The model under review builds one solid part; all positions refer to its coordinate system, in mm. Face numbers are marked on the shaded views. A direction names the side the tool comes from. Give positions to 0.01 mm unless a question says otherwise; leave off trailing zeros. Order: outer loops, then holes, each group sorted by start corner. A loop starts at its lowest first (then second) coordinate and runs counter-clockwise, first axis right, second up.
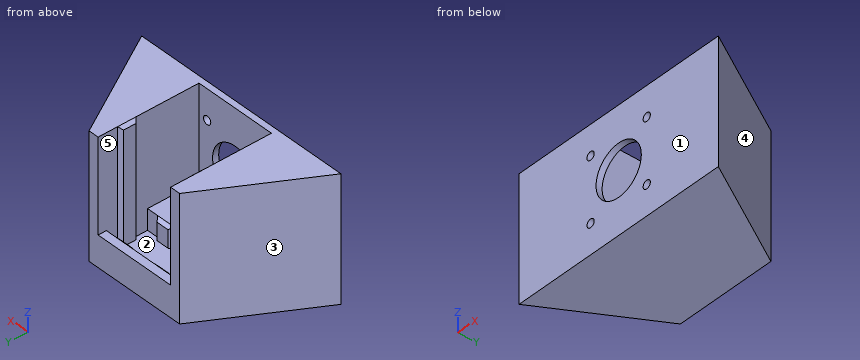
```python
from build123d import *

# Parameters (mm, degrees)
F1_DEPTH  = 60
F2_W      = 40
F2_H      = 20
F3_DEPTH  = 55
F4_W      = 40
F4_H      = 45
F5_DEPTH  = 4
F6_W      = 40
F6_H      = 45
F7_DEPTH  = 25
F8_R      = 12.5
F8_R_2    = 2
F9_DEPTH  = 2.9615242271
F10_W     = 9
F10_H     = 1.5
F10_W_2   = 1.5
F10_H_2   = 9
F11_DEPTH = 10
F12_DEPTH = 45
F13_SIZE  = 1.49999


# Not quite as in the source:
# - a fillet or chamfer is up to 0.001 mm smaller than in the source, because OpenCascade refuses the exact size


with BuildPart() as f1:
    # F0 (on Top) → F1 (new body)
    with BuildSketch(Plane.XY):
        Polygon((30, 51.9615242271), (0, 0), (110, 0), (80, 51.9615242271), align=None)
    extrude(amount=F1_DEPTH)

    # F2 (on face) → F3 (cut)
    with BuildSketch(Plane.XY.offset(60)):
        with Locations((55, 37.9615242271)):
            Rectangle(F2_W, F2_H)
    extrude(amount=-F3_DEPTH, mode=Mode.SUBTRACT)

    # F4 (on face) → F5 (cut, through all)
    with BuildSketch(Plane(origin=(0, 51.9615242271, 0), x_dir=(-1, 0, 0), z_dir=(0, 1, 0))):
        with Locations((-55, 37.5)):
            Rectangle(F4_W, F4_H)
    extrude(amount=-F5_DEPTH, mode=Mode.SUBTRACT)

    # F6 (on face) → F7 (cut)
    with BuildSketch(Plane(origin=(0, 27.9615242271, 0), x_dir=(-1, 0, 0), z_dir=(0, 1, 0))):
        with Locations((-55, 37.5)):
            Rectangle(F6_W, F6_H)
    extrude(amount=-F7_DEPTH, mode=Mode.SUBTRACT)

    # F8 (on face) → F9 (cut, through all)
    with BuildSketch(Plane.XZ):
        with Locations((55, 30)):
            Circle(F8_R)
        with Locations((70.5, 45.5)):
            Circle(F8_R_2)
        with Locations((39.5, 45.5)):
            Circle(F8_R_2)
        with Locations((39.5, 14.5)):
            Circle(F8_R_2)
        with Locations((70.5, 14.5)):
            Circle(F8_R_2)
    extrude(amount=-F9_DEPTH, mode=Mode.SUBTRACT)

    # F10 (on face) → F11 (join, through all)
    with BuildSketch(Plane.XY.offset(15)):
        with Locations((45, 47.2115242271)):
            Rectangle(F10_W, F10_H)
        with Locations((65, 47.2115242271)):
            Rectangle(F10_W, F10_H)
        with Locations((45, 28.7115242271)):
            Rectangle(F10_W, F10_H)
        with Locations((65, 28.7115242271)):
            Rectangle(F10_W, F10_H)
        with Locations((35.75, 37.9615242271)):
            Rectangle(F10_W_2, F10_H_2)
        with Locations((74.25, 37.9615242271)):
            Rectangle(F10_W_2, F10_H_2)
    extrude(amount=-F11_DEPTH)

    # F12 (add, through all): faces of the model
    f12_faces = [f1.faces().sort_by_distance(p)[0] for p in [
        (74.25, 37.9615242271, 15),
        (35.75, 37.9615242271, 15),
    ]]
    extrude(f12_faces, amount=F12_DEPTH)

    # F13 (size 1.5 in the source; OpenCascade refuses exactly that, so slightly less here)
    f13_edges = [f1.edges().sort_by_distance(p)[0] for p in [
        (36.5, 33.461524, 32.5),
        (73.5, 37.961524, 60),
        (73.5, 42.461524, 32.5),
        (36.5, 37.961524, 60),
        (36.5, 42.461524, 32.5),
        (73.5, 33.461524, 32.5),
        (65, 29.461524, 15),
        (69.5, 29.461524, 10),
        (60.5, 29.461524, 10),
        (49.5, 29.461524, 10),
        (45, 29.461524, 15),
        (40.5, 46.461524, 10),
        (45, 46.461524, 15),
        (60.5, 46.461524, 10),
        (65, 46.461524, 15),
        (49.5, 46.461524, 10),
        (40.5, 29.461524, 10),
        (69.5, 46.461524, 10),
    ]]
    chamfer(f13_edges, length=F13_SIZE)


solid = f1.part
```
Item 1: Clearance check with flat-ended pins moving along their axes: pin 1 Ø3.5 at (x, z) = (39.5, 45.5) entering from +Y; pin 2 Ø12 at (x, z) = (12, 34) entering from -Y; pin 3 Ø6 at (x, z) = (57.5, 54) entering from +Y; pin 4 Ø12 at (y, z) = (14.5, 31) entering from -X. State where each tip first meets the part, or that it passes through.
Values found:
pin 1: passes through
pin 2: stops at y = 0
pin 3: stops at y = 2.96
pin 4: stops at x = 4.91
Item 2: For the marked faces 4 and 5, list the 3-axis set-ups (+Z, -Z, +X, -X, +Y, -Y) from which the entire face can be reached by the end or side of a thin tool; tool diameter is ignored.
Values found:
face 4: +Z, -Z, +X, +Y
face 5: +Z
Item 3: Take a section at B-B (x = 55). Give the boundary of the cut face in (y, z), and give its area (3 significant figures).
Values found:
outline: (0, 0) - (51.96, 0) - (51.96, 15) - (47.96, 15) - (47.96, 5) - (27.96, 5) - (27.96, 15) - (2.96, 15) - (2.96, 17.5) - (0, 17.5) - close; (0, 42.5) - (2.96, 42.5) - (2.96, 60) - (0, 60) - close
area: 639 mm2
Item 4: For line 1 (Z direction, x = 70.5, y = 2.05); line 2 (X direction, y = 1, z = 14); line 3 (Y direction, x = 67.5, z = 15.5), list the stretches that pass through material, from the lowest coordinate up.
Values found:
line 1: z = 0 to 12.5, 16.5 to 43.5, 47.5 to 60
line 2: x = 0.58 to 37.56, 41.44 to 68.56, 72.44 to 109.42
line 3: y = 0 to 2.96
Item 5: Draft analysis for pull direction X (two halves, no side actions). For the marked faces 1, 2 and 3, state which applies: released by +X, released by -X, zero draft, split by the parting line, or undercut.
Values found:
face 1: zero draft
face 2: undercut
face 3: released by -X
Item 6: Take a section at A-A (z = 45.5). Give the number of separate pieces and of enclosed holes in the cut face, and give its area (3 significant figures).
Values found:
separate pieces: 3
enclosed holes: 0
area: 2,200 mm2
